Can you work these out from the model? Positions are in its coordinate system, mm. A direction names the side the tool comes from. Round coordinates to 2 decimals unless told otherwise and drop trailing zeros. Loops run counter-clockwise (first coordinate to the right, second up) from the corner with the lowest first, then second, coordinate; pieces in that order, holes last. Notation, with made-up numbers: (84, 5) -> (136, 5) arc R18 cw to (136, 30) -> close; hole circle Ø5 at (67.5, -29). An arc over 180 degrees is marked (long way). Answer as a JSON object with one key per item and string values.
```python
from build123d import *

# Parameters (mm, degrees)
SKETCH_1_W          = 35
SKETCH_1_H          = 4
EXTRUDE_1_DEPTH     = 25
CHAMFER_1_SIZE      = 1.5
SKETCH_2_W          = 12.744138526
SKETCH_2_H          = 17.309109507
CUT_EXTRUDE_1_DEPTH = 10


with BuildPart() as part:
    # 草图1 → 凸台-拉伸1 (new body)
    with BuildSketch(Plane(origin=(0, 0, 0), x_dir=(1, 0, 0), z_dir=(0, 1, 0))):
        Rectangle(SKETCH_1_W, SKETCH_1_H)
    extrude(amount=EXTRUDE_1_DEPTH)

    # 倒角1
    chamfer_1_edges = [part.edges().sort_by_distance(p)[0] for p in [
        (0, 0, 2),
        (0, 0, -2),
    ]]
    chamfer(chamfer_1_edges, length=CHAMFER_1_SIZE)

    # 草图2 → 切除-拉伸1 (cut)
    with BuildSketch(Plane(origin=(0, 0, -2), x_dir=(-1, 0, 0), z_dir=(0, 0, -1))):
        with Locations((-1.305884938, 6.001185717)):
            Rectangle(SKETCH_2_W, SKETCH_2_H)
    extrude(amount=-CUT_EXTRUDE_1_DEPTH, mode=Mode.SUBTRACT)


solid = part.part
```
Q1. I want a section at B-B, the plane z = -1.4. Write out the boundary of the cut face in (x, y), then the cut area to 3 significant figures.
Determined:
{"outline": "(-17.5, 0.9) -> (-5.07, 0.9) -> (-5.07, 14.66) -> (7.68, 14.66) -> (7.68, 0.9) -> (17.5, 0.9) -> (17.5, 25) -> (-17.5, 25) -> close", "area": "668 mm²"}
Q2. I want a section at A-A, the plane y = 4.25. Write out the boundary of the cut face in (x, z), then the cut area to 3 significant figures.
Determined:
{"outline": "(-17.5, -2) -> (-5.07, -2) -> (-5.07, 2) -> (-17.5, 2) -> close; (7.68, -2) -> (17.5, -2) -> (17.5, 2) -> (7.68, 2) -> close", "area": "89.0 mm²"}
Q3. We'd pull the mould along X, two halves only. Please class faces 3 (the flat face through (17.5, 12, 0)), 4 (the flat face through (13, 0, 0)), 5 (the flat face through (1, 14.656, 0)): pulls with the +X half, pulls with the -X half, needs draft (parallel to the pull), parting line crosses it, or undercut.
Determined:
{"face 3": "pulls with the +X half", "face 4": "needs draft", "face 5": "undercut"}
Q4. On a 3-axis mill with a long thin cutter (end or side, diameter ignored), from which of +Z, -Z, +X, -X, +Y, -Y can I reach the whole of each face in a straight line? I mean faces 1 (the flat face through (0, 25, 0)), 2 (the flat face through (-5.066, 7, 0)). Say none if no direction works.
Determined:
{"face 1": "+Z, -Z, +X, -X, +Y", "face 2": "+Z, -Z, -Y"}
Q5. I want a section at D-D, the plane x = 5.5. Write out the boundary of the cut face in (y, z), then the cut area to 3 significant figures.
Determined:
{"outline": "(14.66, -2) -> (25, -2) -> (25, 2) -> (14.66, 2) -> close", "area": "41.4 mm²"}
Q6. If I drill on L1, parallel to X at y = 8.25, z = 1.85; L2, parallel to Y at x = -5, z = 1.05; L3, parallel to Y at x = -8, z = 1.85, over which ranges is the centre line in solid material (lowest first)? Write a range as [from, to].
Determined:
{"L1": "[-17.5, -5.07], [7.68, 17.5]", "L2": "[14.66, 25]", "L3": "[1.35, 25]"}
Q7. I'm going to push a flat-ended pin straight in: pin 1 (1.2 mm diameter, centred on x = 0, z = 1, fed in from -Y). Where does the tip first touch, or does it pass through?
Determined:
{"pin 1": "y = 14.66"}
Q8. I want a section at C-C, the plane x = 9. Write out the boundary of the cut face in (y, z), then the cut area to 4 significant figures.
Determined:
{"outline": "(0, -0.5) -> (1.5, -2) -> (25, -2) -> (25, 2) -> (1.5, 2) -> (0, 0.5) -> close", "area": "97.75 mm²"}
